Part model, mm, in its own coordinate system. A direction names the side the tool comes from. Coordinates: 2 decimals unless noted, no trailing zeros. Write each loop counter-clockwise with the first axis right and the second up, starting at its lowest first coordinate (ties: lowest second). Pieces come first, ordered by that corner, then holes. Notation, with made-up numbers: (21.25, 29.25) - (56.25, 29.25) arc R28 ccw to (56.25, 57.25) - close; hole circle Ø11 at (-17.5, -23.5). An arc over 180 degrees is marked (long way). Use a Markdown table: item, result.
```python
from build123d import *

# Parameters (mm, degrees)
F0_W     = 409.575
F0_H     = 85.725
F0_W_2   = 9.525
F0_H_2   = 41.275
F1_DEPTH = 19.05
F2_DEPTH = 4.7625


with BuildPart() as f1:
    # F0 (on Front) → F1 (new body)
    with BuildSketch(Plane.XZ):
        Rectangle(F0_W, F0_H)
        with Locations((-161.925, -12.7)):
            Rectangle(F0_W_2, F0_H_2, mode=Mode.SUBTRACT)
        with Locations((161.925, -12.7)):
            Rectangle(F0_W_2, F0_H_2, mode=Mode.SUBTRACT)
        with Locations((161.925, -12.7)):
            Rectangle(F0_W_2, F0_H_2)
        with Locations((-161.925, -12.7)):
            Rectangle(F0_W_2, F0_H_2)
    extrude(amount=F1_DEPTH)

    # F0 (on Front) → F2 (cut)
    with BuildSketch(Plane.XZ):
        with Locations((161.925, -12.7)):
            Rectangle(F0_W_2, F0_H_2)
        with Locations((-161.925, -12.7)):
            Rectangle(F0_W_2, F0_H_2)
    extrude(amount=F2_DEPTH, mode=Mode.SUBTRACT)


solid = f1.part
```
Item 1: Drop flat-ended pins along their axis: P1, Ø7.5, axis at x = 161, z = -9, coming from the +Y side; P2, Ø8, axis at x = 130, z = 24, coming from the +Y side. Give the stop position or say it passes through.
From the geometry:
| item | result |
|---|---|
| P1 | y = -4.76 |
| P2 | y = 0 |
Item 2: Drill centre lines: probe 1 along X at (y, z) = (-1.5, -5); probe 2 along Z at (x, y) = (161.5, -3.5). Where is each one in solid material? Low to high.
From the geometry:
| item | result |
|---|---|
| probe 1 | -204.79 to -166.69, -157.16 to 157.16, 166.69 to 204.79 |
| probe 2 | -42.86 to -33.34, 7.94 to 42.86 |
Item 3: Band-saw the part on A-A, the plane x = 161. Give the cut face in (y, z), then the cut area to 3 significant figures.
From the geometry:
| item | result |
|---|---|
| outline | (-19.05, -42.86) - (0, -42.86) - (0, -33.34) - (-4.76, -33.34) - (-4.76, 7.94) - (0, 7.94) - (0, 42.86) - (-19.05, 42.86) - close |
| area | 1,440 mm^2 |
Item 4: Two-plate mould, pull along Z, no slides. Class faces 1 (the face through (-162, -4.762, -12)), 2 (the face through (-3, 0, 1)), 3 (the face through (-3, -9, -42.862)): pulls with the +Z half, pulls with the -Z half, needs draft (parallel to the pull), parting line crosses it, or undercut.
From the geometry:
| item | result |
|---|---|
| face 1 | undercut |
| face 2 | needs draft |
| face 3 | pulls with the -Z half |
Item 5: Which spindle directions (+Z, -Z, +X, -X, +Y, -Y) get a long thin tool onto all of the face, cutting with end or side? Do faces 4 (the face through (-3, -9, 42.862)), 5 (the face through (162, -4.762, -12)). Say none if no direction does.
From the geometry:
| item | result |
|---|---|
| face 4 | +Z, +X, -X, +Y, -Y |
| face 5 | +Y |
